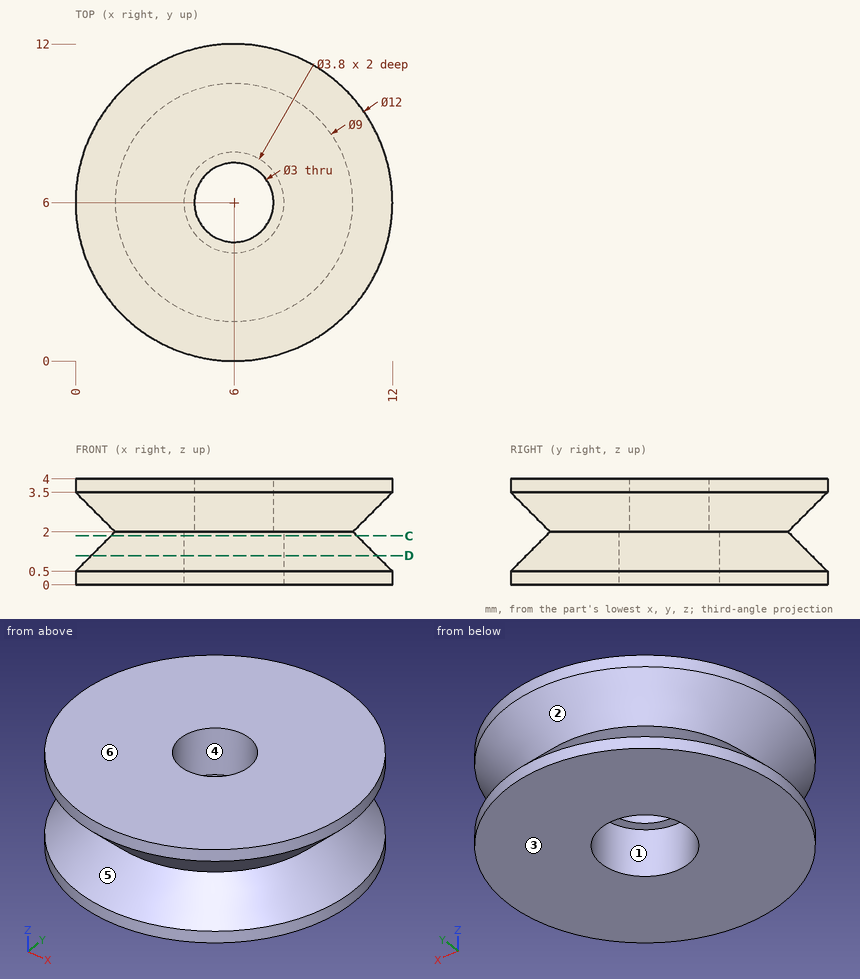
Drawing for the job (mm, zero at the part's lowest x, y, z). A direction names the side the tool comes from. Give positions to 0.01 mm unless a question says otherwise; leave off trailing zeros. Loops run counter-clockwise (first coordinate to the right, second up) from the corner with the lowest first, then second, coordinate; pieces in that order, holes last. Notation, with made-up numbers: M -2,28 L 6,28 A17 cw 6,49 Z; hole C 68.5,88.25 d9. An arc over 180 degrees is marked long. Use one line per item in the form item = value.
Item 1: Two-plate mould, pull along X, no slides. Class the marked faces 4, 5 and 6: pulls with the +X half, pulls with the -X half, needs draft (parallel to the pull), parting line crosses it, or undercut.
Determined:
face_4 = undercut
face_5 = parting line crosses it
face_6 = needs draft
Item 2: Flat gauge pins, fed straight in: pin 1 (1.8 mm diameter, centred on x = 6, y = 6, fed in from +Z); pin 2 (1 mm diameter, centred on x = 7.5, z = 2, fed in from -Y). Where does each tip first touch, or does it go through?
Determined:
pin_1 = through
pin_2 = 1.21
Item 3: Drill centre lines: probe 1 along Y at (x, z) = (6, 3.55); probe 2 along Y at (x, z) = (6, 2.95); probe 3 along Z at (x, y) = (9.25, 9.25). Where is each one in solid material? Low to high. Write a range as from..to.
Determined:
probe_1 = 0..4.5, 7.5..12
probe_2 = 0.55..4.5, 7.5..11.45
probe_3 = 0..1.9, 2.1..4
Item 4: Which spindle directions (+Z, -Z, +X, -X, +Y, -Y) get a long thin tool onto all of the face, cutting with end or side? Do the marked faces 1, 2 and 3. Say none if no direction does.
Determined:
face_1 = -Z
face_2 = none
face_3 = -Z, +X, -X, +Y, -Y
Item 5: Slice it at C-C (z = 1.85). List the corners of the cut face in (x, y).
Determined:
outline = C 6,6 d9.3; hole C 6,6 d3.8
Item 6: Slice it at D-D (z = 1.1). List the corners of the cut face in (x, y).
Determined:
outline = C 6,6 d10.8; hole C 6,6 d3.8
